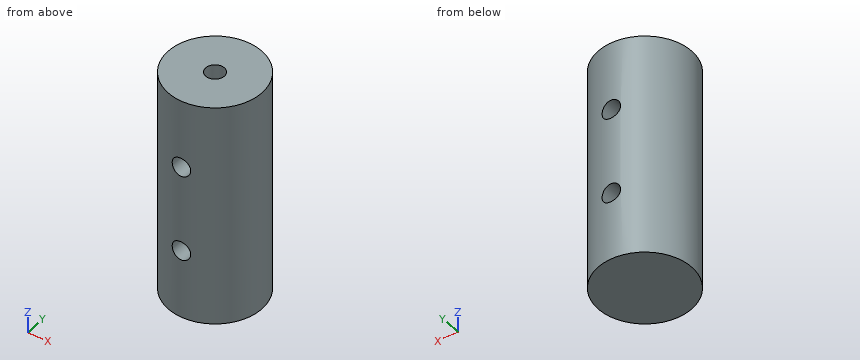
from build123d import *

# Parameters (mm, degrees)
F0_R     = 15.875
F1_DEPTH = 76.2
F2_R     = 3.175
F3_DEPTH = 63.5
F4_R     = 3.175
F5_DEPTH = 25.4


with BuildPart() as f1:
    # F0 (on Top) → F1 (new body)
    with BuildSketch(Plane.XY):
        Circle(F0_R)
    extrude(amount=F1_DEPTH)

    # F2 (on face) → F3 (cut)
    with BuildSketch(Plane.XY.offset(76.2)):
        Circle(F2_R)
    extrude(amount=-F3_DEPTH, mode=Mode.SUBTRACT)

    # F4 (on Front) → F5 (cut, symmetric)
    with BuildSketch(Plane.XZ):
        with Locations((0, 23.36292)):
            Circle(F4_R)
        with Locations((0, 52.832)):
            Circle(F4_R)
    extrude(amount=F5_DEPTH, both=True, mode=Mode.SUBTRACT)


solid = f1.part
Work out the finished part from the listing and answer in its coordinate system (mm). Give positions to 0.01 mm unless a question says otherwise; leave off trailing zeros. Loops run counter-clockwise (first coordinate to the right, second up) from the corner with the lowest first, then second, coordinate; pieces in that order, holes last. Notation, with made-up numbers: M 26,-21 L 35,-21 A31 cw 35,14 Z; hole C 24,64.5 d5. An arc over 180 degrees is marked long. Use CSV: the item, a comma, the result in double quotes.
1) Find section C-C on z = 47.5. Write down the section's boundary in (x, y) (3 decimals).
Answer:
outline,"C 0,0 d31.75; hole C 0,0 d6.35"
2) Consider L1, parallel to Z at x = 0, y = 8.5; L2, parallel to Y at x = 0, z = 16.75 (3 decimals); L3, parallel to Z at x = -1, y = 9. Determine where each line is inside the solid, lowest interval first.
Answer:
L1,"0 to 20.19, 26.54 to 49.66, 56.01 to 76.2"
L2,"-15.875 to -3.175, 3.175 to 15.875"
L3,"0 to 20.35, 26.38 to 49.82, 55.85 to 76.2"
3) Find section A-A on x = 0. Write down the section's boundary in (y, z) (3 decimals).
Answer:
outline,"M -15.875,0 L 15.875,0 L 15.875,20.188 L 3.175,20.188 L 3.175,12.7 L -3.175,12.7 L -3.175,20.188 L -15.875,20.188 Z; M -15.875,26.538 L -3.175,26.538 L -3.175,49.657 L -15.875,49.657 Z; M -15.875,56.007 L -3.175,56.007 L -3.175,76.2 L -15.875,76.2 Z; M 3.175,26.538 L 15.875,26.538 L 15.875,49.657 L 3.175,49.657 Z; M 3.175,56.007 L 15.875,56.007 L 15.875,76.2 L 3.175,76.2 Z"
4) Find section B-B on y = 8. Write down the section's boundary in (x, z) (3 decimals).
Answer:
outline,"M -13.712,0 L 13.712,0 L 13.712,76.2 L -13.712,76.2 Z; hole C 0,23.363 d6.35; hole C 0,52.832 d6.35"
5) Find section D-D on x = 11.5. Write down the section's boundary in (y, z).
Answer:
outline,"M -10.94,0 L 10.94,0 L 10.94,76.2 L -10.94,76.2 Z"
6) Given P1, Ø1, axis at y = -3.5, z = 34, coming from the +X side; P2, Ø5.5, axis at x = 0, y = 0, coming from the -Z side; P3, Ø5.5, axis at x = 0, z = 23.36, coming from the +Y side; P4, Ø6, axis at y = -9.5, z = 20.5, coming from the -X side, each flat-ended and moving along its own axis, determine where each tip first touches the part or whether it passes through.
Answer:
P1,"x = 15.59"
P2,"z = 0"
P3,"through"
P4,"x = -14.48"
